Check sheet for the modelled part. Datum: model origin and axes. Units: mm. A direction names the side the tool comes from. Round coordinates to 2 decimals unless told otherwise and drop trailing zeros. Order: outer loops, then holes, each group sorted by start corner. A loop starts at its lowest first (then second) coordinate and runs counter-clockwise, first axis right, second up.
Q1. Set-up check for faces 1 (the flat face through (-62, -18.95, -3)), 2 (the flat face through (-20, -8, -9.333)), 3 (the flat face through (-6.982, -7, -6)): record each of +Z, -Z, +X, -X, +Y, -Y from which the full face is reachable in a straight line by a thin tool's end or side.
Q2. Cross-section at B-B on y = -25. Record the cut outline in (x, z), then the cut area to 3 significant figures.
Q3. Cross-section at A-A on z = -7.5. Record the cut outline in (x, y).
Q4. Mould release check, pull along X, two halves, no side actions. Record for faces 4 (the flat face through (-30.25, -7, -6)), 5 (the flat face through (-20, -8, -2.845)), 6 (the flat face through (-20, -7, -10.7)), 7 (the flat face through (58.825, -19, 2)): +X half, -X half, draft (parallel to the pull), parting line (faces both ways), or undercut.
Q5. Cross-section at D-D on x = 5. Record the cut outline in (y, z).
Q6. Cross-section at C-C on y = 17.5. Record the cut outline in (x, z) (3 decimals), then the cut area to 3 significant figures.
Q7. Scan lines: probe 1 along Z at (x, y) = (-55, -18); probe 2 along X at (y, z) = (17, -1); probe 3 along Z at (x, y) = (-17, -22.5). Record each from-to range of solid material in increasing order.
Q8. Depth check by flat-ended pin: P1, Ø2.5, axis at x = -72.425, y = 25, coming from the +Z side; P2, Ø2.5, axis at x = -62.5, z = -3, coming from the -Y side; P3, Ø7, axis at y = -9, z = -5, coming from the +X side; P4, Ø9.5, axis at y = -8.5, z = -6.5, coming from the +X side. Enter the tip coordinate at first touch or a pass-through.
from build123d import *

# Parameters (mm, degrees)
SKETCH1_W                = 150.5
SKETCH1_H                = 55.1
SKETCH1_R                = 1.575
SKETCH1_R_2              = 6.5
SKETCH1_W_2              = 12.1
SKETCH1_H_2              = 12.1
SKETCH1_W_3              = 6
SKETCH1_H_3              = 6
BOSS_EXTRUDE1_DEPTH      = 1.7
SKETCH3_W                = 12.1
SKETCH3_H                = 12.1
BOSS_EXTRUDE2_DEPTH      = 4.25
BOSS_EXTRUDE2_DEPTH_BACK = 1.7
SKETCH5_R                = 3
BOSS_EXTRUDE3_DEPTH      = 20
CUT_EXTRUDE1_DEPTH       = 9.4
SKETCH7_W                = 6
SKETCH7_H                = 6
BOSS_EXTRUDE4_DEPTH      = 3.6
BOSS_EXTRUDE4_DEPTH_BACK = 1.7
SKETCH8_R                = 1.7
BOSS_EXTRUDE5_DEPTH      = 0.6
SKETCH9_W                = 26.4
SKETCH9_H                = 26.6
BOSS_EXTRUDE6_DEPTH      = 2.75
BOSS_EXTRUDE7_DEPTH      = 26.6
SKETCH11_W               = 2.263245578
SKETCH11_H               = 25.200228651
CUT_EXTRUDE2_DEPTH       = 25.75
SKETCH12_W               = 20.23176928
SKETCH12_H               = 8.8
SKETCH12_W_2             = 20.955499341
BOSS_EXTRUDE8_DEPTH      = 9
SKETCH13_W               = 17.717825076
SKETCH13_H               = 6.488260173
SKETCH13_W_2             = 18.921956069
CUT_EXTRUDE3_DEPTH       = 8


with BuildPart() as part:
    # Sketch1 → Boss-Extrude1 (new body)
    with BuildSketch(Plane.XY):
        Rectangle(SKETCH1_W, SKETCH1_H)
        with Locations((-72.425, 25)):
            Circle(SKETCH1_R, mode=Mode.SUBTRACT)
        with Locations((72.425, 25)):
            Circle(SKETCH1_R, mode=Mode.SUBTRACT)
        with Locations((72.425, -25)):
            Circle(SKETCH1_R, mode=Mode.SUBTRACT)
        with Locations((-72.425, -25)):
            Circle(SKETCH1_R, mode=Mode.SUBTRACT)
        with Locations((61.825, 17.5)):
            Circle(SKETCH1_R_2, mode=Mode.SUBTRACT)
        with Locations((61.825, -2)):
            Rectangle(SKETCH1_W_2, SKETCH1_H_2, mode=Mode.SUBTRACT)
        with Locations((61.825, -19)):
            Rectangle(SKETCH1_W_3, SKETCH1_H_3, mode=Mode.SUBTRACT)
    extrude(amount=-BOSS_EXTRUDE1_DEPTH)

    # Sketch3 → Boss-Extrude2 (add, two sides)
    with BuildSketch(Plane.XY) as boss_extrude2_sk:
        with Locations((61.825, -2)):
            Rectangle(SKETCH3_W, SKETCH3_H)
    extrude(amount=BOSS_EXTRUDE2_DEPTH)
    extrude(boss_extrude2_sk.sketch, amount=-BOSS_EXTRUDE2_DEPTH_BACK)

    # Sketch5 → Boss-Extrude3 (add)
    with BuildSketch(Plane.XY.offset(4.25)):
        with Locations((61.825, -2)):
            Circle(SKETCH5_R)
    extrude(amount=BOSS_EXTRUDE3_DEPTH)

    # Sketch6 → Cut-Extrude1 (cut)
    with BuildSketch(Plane.XY.offset(24.25)):
        Polygon((61.825, 1), (64.333206892, -3.645873077), (66.484499698, -3.318483035), (63.123279269, 3.423164798), align=None)
    extrude(amount=-CUT_EXTRUDE1_DEPTH, mode=Mode.SUBTRACT)

    # Sketch7 → Boss-Extrude4 (add, two sides)
    with BuildSketch(Plane.XY) as boss_extrude4_sk:
        with Locations((61.825, -19)):
            Rectangle(SKETCH7_W, SKETCH7_H)
    extrude(amount=BOSS_EXTRUDE4_DEPTH)
    extrude(boss_extrude4_sk.sketch, amount=-BOSS_EXTRUDE4_DEPTH_BACK)

    # Sketch8 → Boss-Extrude5 (add)
    with BuildSketch(Plane.XY.offset(3.6)):
        with Locations((61.825, -19)):
            Circle(SKETCH8_R)
    extrude(amount=BOSS_EXTRUDE5_DEPTH)

    # Sketch9 → Boss-Extrude6 (add)
    with BuildSketch(Plane(origin=(0, 0, -1.7), x_dir=(-1, 0, 0), z_dir=(0, 0, -1))):
        with Locations((62.05, -5.65)):
            Rectangle(SKETCH9_W, SKETCH9_H)
    extrude(amount=BOSS_EXTRUDE6_DEPTH)

    # Sketch10 → Boss-Extrude7 (add)
    with BuildSketch(Plane(origin=(0, 7.65, 0), x_dir=(1, 0, 0), z_dir=(0, 1, 0))):
        Polygon((-75.25, 4.45), (-75.25, 4.95), (-73.05, 4.45), align=None)
    extrude(amount=-BOSS_EXTRUDE7_DEPTH)

    # Sketch11 → Cut-Extrude2 (cut)
    with BuildSketch(Plane.ZY.offset(75.25)):
        with Locations((-3.161622789, -5.606749437)):
            Rectangle(SKETCH11_W, SKETCH11_H)
    extrude(amount=-CUT_EXTRUDE2_DEPTH, mode=Mode.SUBTRACT)

    # Sketch12 → Boss-Extrude8 (add)
    with BuildSketch(Plane(origin=(0, 0, -1.7), x_dir=(-1, 0, 0), z_dir=(0, 0, -1))):
        with Locations((-3.13411536, -7.1)):
            Rectangle(SKETCH12_W, SKETCH12_H)
        with Locations((19.77225033, -7.1)):
            Rectangle(SKETCH12_W_2, SKETCH12_H)
    extrude(amount=BOSS_EXTRUDE8_DEPTH)

    # Sketch13 → Cut-Extrude3 (cut)
    with BuildSketch(Plane.XZ.offset(11.5)):
        with Locations((3.496108, -6.088951298)):
            Rectangle(SKETCH13_W, SKETCH13_H)
        with Locations((-19.500417756, -6.088951298)):
            Rectangle(SKETCH13_W_2, SKETCH13_H)
    extrude(amount=-CUT_EXTRUDE3_DEPTH, mode=Mode.SUBTRACT)


solid = part.part
Results found:
1. face 1: -Z, +X, -X, -Y
1. face 2: -Y
1. face 3: -Z, +Y, -Y
2. outline: (-75.25, -1.7) - (-74, -1.7) - (-74, 0) - (-75.25, 0) - close; (-70.85, -1.7) - (70.85, -1.7) - (70.85, 0) - (-70.85, 0) - close; (74, -1.7) - (75.25, -1.7) - (75.25, 0) - (74, 0) - close
2. area: 245 mm2
3. outline: (-30.25, -11.5) - (-28.96, -11.5) - (-28.96, -3.5) - (-10.04, -3.5) - (-10.04, -11.5) - (-9.29, -11.5) - (-9.29, -2.7) - (-30.25, -2.7) - close; (-6.98, -11.5) - (-5.36, -11.5) - (-5.36, -3.5) - (12.36, -3.5) - (12.36, -11.5) - (13.25, -11.5) - (13.25, -2.7) - (-6.98, -2.7) - close
4. face 4: undercut
4. face 5: undercut
4. face 6: draft
4. face 7: -X half
5. outline: (-27.55, -1.7) - (-11.5, -1.7) - (-11.5, -2.84) - (-3.5, -2.84) - (-3.5, -9.33) - (-11.5, -9.33) - (-11.5, -10.7) - (-2.7, -10.7) - (-2.7, -1.7) - (27.55, -1.7) - (27.55, 0) - (-27.55, 0) - close
6. outline: (-75.25, -1.7) - (55.325, -1.7) - (55.325, 0) - (-75.25, 0) - close; (68.325, -1.7) - (75.25, -1.7) - (75.25, 0) - (68.325, 0) - close
6. area: 234 mm2
7. probe 1: z = -4.45 to -4.29, -2.03 to 0
7. probe 2: x = -75.25 to 55.34, 68.31 to 75.25
7. probe 3: z = -1.7 to 0
8. P1: passes through
8. P2: stops at y = -18.95
8. P3: stops at x = 75.25
8. P4: stops at x = 13.25
